Check sheet for the modelled part. Datum: model origin and axes. Units: mm. Round coordinates to 2 decimals unless told otherwise and drop trailing zeros. One line per question, with ' | ' between items.
```python
from build123d import *

# Parameters (mm, degrees)
F2_R = 5
F3_R = 70


with BuildPart() as f1:
    # F0 (on Top) → F1 (revolve)
    with BuildSketch(Plane.XY):
        Polygon((-25, 0), (-25, 9.5), (-29, 13.5), (-45, 13.5), (-49, 9.5), (-50, 0), (-49, -9.5), (-45, -13.5), (-29, -13.5), (-25, -9.5), align=None)
        Polygon((-25, 0), (-25, 9.5), (-29, 13.5), (-45, 13.5), (-49, 9.5), (-50, 0), (-49, -9.5), (-45, -13.5), (-29, -13.5), (-25, -9.5), align=None)
    revolve(axis=Axis((0, 18.855867, 0), (0, 1, 0)))

    # F2
    f2_edges = [f1.edges().sort_by_distance(p)[0] for p in [
        (29, -13.5, 0),
        (45, -13.5, 0),
        (49, -9.5, 0),
        (45, 13.5, 0),
        (29, 13.5, 0),
        (49, 9.5, 0),
    ]]
    fillet(f2_edges, radius=F2_R)

    # F3
    f3_edges = [f1.edges().sort_by_distance(p)[0] for p in [
        (50, 0, 0),
    ]]
    fillet(f3_edges, radius=F3_R)


solid = f1.part
```
(1) Mould release check, pull along X, two halves, no side actions. Record for faces 1 (the face through (22.1, 13.5, 22.5)), 2 (the face through (5.45, 9.66, -24.56)): +X half, -X half, draft (parallel to the pull), parting line (faces both ways), or undercut.
Answer:
face 1: draft | face 2: undercut
(2) Go/stop test with flat-tipped pins: pin 1 (10 mm diameter, centred on x = -12.5, y = -9, fed in from +Z); pin 2 (1.5 mm diameter, centred on x = 10.5, y = -0.5, fed in from -Z); pin 3 (10 mm diameter, centred on y = 9, z = 29.5, fed in from +X). Record where each tip stops, or that it passes through.
Answer:
pin 1: stops at z = 48.63 | pin 2: stops at z = -48.64 | pin 3: stops at x = 42.56
(3) Scan lines: probe 1 along X at (y, z) = (-2.75, 17); probe 2 along Z at (x, y) = (0, 2.25); probe 3 along Z at (x, y) = (0, -3.5). Record each from-to range of solid material in increasing order.
Answer:
probe 1: x = -46.55 to -18.33, 18.33 to 46.55 | probe 2: z = -49.58 to -25, 25 to 49.58 | probe 3: z = -49.53 to -25, 25 to 49.53
